The model under review builds one solid part; all positions refer to its coordinate system, in mm. Face numbers are marked on the shaded views. Round coordinates to 2 decimals unless told otherwise and drop trailing zeros. Order: outer loops, then holes, each group sorted by start corner. A loop starts at its lowest first (then second) coordinate and runs counter-clockwise, first axis right, second up.
1) Consider section D-D (x = 1). Give the boundary of the cut face in (y, z).
2) Mouldability with a two-part tool opening along X and no side actions: class the marked faces 1, 2 and 3 as pulls with the +X half, pulls with the -X half, needs draft (parallel to the pull), parting line crosses it, or undercut.
3) Consider section B-B (x = 5). Give the boundary of the cut face in (y, z), then the cut area to 3 significant figures.
4) To check wall thickness, follow L1, parallel to Z at x = 5, y = 3; L2, parallel to Z at x = 6, y = 4.75; L3, parallel to Y at x = 11, z = 10. State the ranges of each line that lie inside material, in increasing order.
5) Consider section A-A (y = 5). Give the boundary of the cut face in (x, z), then the cut area to 3 significant figures.
6) Clearance check with a flat-ended pin moving along its axis: P1, Ø2, axis at x = 3, z = 11, coming from the -Y side. State where the tip first meets the part, or that it passes through.
7) Consider section C-C (z = 10). Give the boundary of the cut face in (x, y).
Autodesk Inventor part; units mm, degrees
ref_plane "YZ Plane" through (0, 0, 0) normal (1, 0, 0) x (0, 1, 0)
ref_plane "XZ Plane" through (0, 0, 0) normal (0, 1, 0) x (-1, 0, 0)
ref_plane "XY Plane" through (0, 0, 0) normal (0, 0, 1) x (1, 0, 0)
sketch "Sketch1" plane through (0, 0, 0) normal (0, 0, 1) x (1, 0, 0)
  line L0 (0, 0) -> (15, 0)
  line L1 (15, 0) -> (15, 10)
  line L2 (15, 10) -> (0, 10)
  line L3 (0, 10) -> (0, 0)
  line L4 (1, 9) -> (14, 9)
  line L5 (14, 9) -> (14, 1)
  line L6 (14, 1) -> (1, 1)
  line L7 (1, 1) -> (1, 9)
  dimension "d0" = 15
  dimension "d1" = 10
  dimension "d2" = 13
  dimension "d3" = 8
  dimension "d4" = 1
  dimension "d5" = 1
extrude "Extrusion1" add sketch "Sketch1" along normal blind 20 contours L3 L2 L1 L0 | L4 L5 L6 L7
sketch "Sketch2" plane through (0, 10, 0) normal (0, 1, 0) x (1, 0, 0)
  line L0 (15, 0) -> (0, 0)
  line L1 (0, 0) -> (0, -20)
  line L2 (15, -20) -> (0, -20)
  line L3 (15, 0) -> (15, -20)
  circle A0 centre (5, -5) radius 1.5
  circle A1 centre (5, -15) radius 1.5
  dimension "d8" = 3
  dimension "d9" = 3
  dimension "d10" = 5
  dimension "d11" = 5
  dimension "d12" = 5
  dimension "d13" = 5
extrude "Extrusion2" cut sketch "Sketch2" against normal up to surface (10 mm away) contours A0 | A1
sketch "Sketch3" plane through (15, 0, 0) normal (1, 0, 0) x (0, 0, -1)
  line L0 (0, 0) -> (0, 10)
  line L1 (0, 10) -> (-20, 10)
  line L2 (-20, 0) -> (-20, 10)
  line L3 (0, 0) -> (-20, 0)
  circle A0 centre (-10, 5) radius 1.5
  dimension "d16" = 3
  dimension "d17" = 5
  dimension "d18" = 10
extrude "Extrusion3" cut sketch "Sketch3" against normal up to surface (15 mm away) contours A0
properties part number "profile1"
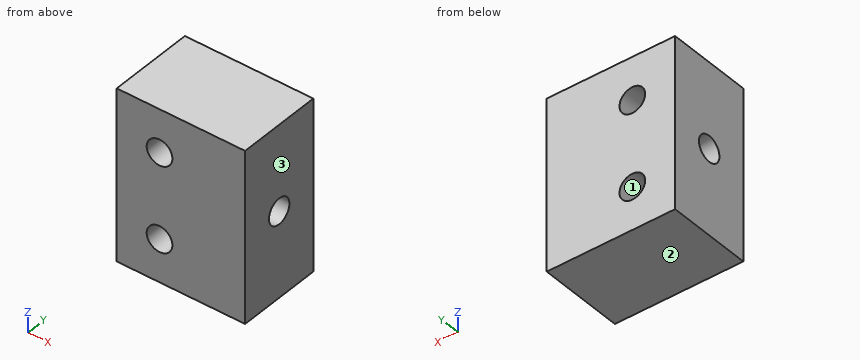
Answer below:
1. outline: (0, 0) - (10, 0) - (10, 20) - (0, 20) - close; hole circle Ø3 at (5, 10)
2. face 1: undercut
2. face 2: needs draft
2. face 3: pulls with the +X half
3. outline: (0, 0) - (10, 0) - (10, 3.5) - (0, 3.5) - close; (0, 6.5) - (10, 6.5) - (10, 13.5) - (0, 13.5) - close; (0, 16.5) - (10, 16.5) - (10, 20) - (0, 20) - close; hole circle Ø3 at (5, 10)
3. area: 133 mm2
4. L1: z = 0 to 3.5, 6.5 to 13.5, 16.5 to 20
4. L2: z = 0 to 3.88, 6.12 to 8.52, 11.48 to 13.88, 16.12 to 20
4. L3: y = 0 to 3.5, 6.5 to 10
5. outline: (0, 0) - (15, 0) - (15, 8.5) - (0, 8.5) - close; (0, 11.5) - (15, 11.5) - (15, 20) - (0, 20) - close; hole circle Ø3 at (5, 5); hole circle Ø3 at (5, 15)
5. area: 241 mm2
6. P1: stops at y = 0
7. outline: (0, 0) - (15, 0) - (15, 3.5) - (0, 3.5) - close; (0, 6.5) - (15, 6.5) - (15, 10) - (0, 10) - close
